The model under review builds one solid part; all positions refer to its coordinate system, in mm. A direction names the side the tool comes from. Give positions to 0.01 mm unless a question says otherwise; leave off trailing zeros. Write each loop counter-clockwise with the first axis right and the second up, starting at its lowest first coordinate (ties: lowest second). Pieces come first, ordered by that corner, then holes. Notation, with made-up numbers: (54, 88.25) -> (82, 88.25) arc R18 cw to (82, 110.25) -> close; hole circle Ø5 at (12.25, 55.25). An arc over 180 degrees is marked (long way). Use CSV: the item, a comma, the result in double quotes.
```python
from build123d import *

# Parameters (mm, degrees)
FASE1_SIZE                                 = 1
F_3_1_3_1_DURCHMESSER_BOHRUNG1_D           = 3.1
F_3_1_3_1_DURCHMESSER_BOHRUNG1_DEPTH       = 15
F_3_1_3_1_DURCHMESSER_BOHRUNG1_CSINK_D     = 3.15
F_3_1_3_1_DURCHMESSER_BOHRUNG1_CSINK_ANGLE = 90
F_3_1_3_1_DURCHMESSER_BOHRUNG1_TIP         = 0.931333959
SCHNITT_LINEAR_AUSTRAGEN1_REACH            = 43.006
SKIZZE5_R                                  = 3
FASE2_SIZE                                 = 1.5


with BuildPart() as part:
    # Skizze1 → Rotation1 (revolve)
    with BuildSketch(Plane.XY, mode=Mode.PRIVATE) as rotation1_sk:
        Polygon((7, 0), (27.5, 0), (27.5, 5.5), (23, 5.5), (23, 6), (19.9, 6), (19.9, 13), (10.6, 13), (10.6, 8), (7, 8), align=None)
    revolve(rotation1_sk.sketch.rotate(Axis((0, 0, 0), (0, -1, 0)), 90), axis=Axis((0, 0, 0), (0, -1, 0)))

    # Fase1
    fase1_edges = [part.edges().sort_by_distance(p)[0] for p in [
        (0, 13, -19.9),
        (0, 13, -10.6),
    ]]
    chamfer(fase1_edges, length=FASE1_SIZE)

    # Ø3.1 (3.1) Durchmesser Bohrung1
    with Locations(Plane(origin=(0, 0, 0), x_dir=(-1, 0, 0), z_dir=(0, -1, 0))):
        with Locations((-16.02146997, 9.25), (0, 18.5), (16.02146997, 9.25), (16.02146997, -9.25), (0, -18.5), (-16.02146997, -9.25)):
            CounterSinkHole(F_3_1_3_1_DURCHMESSER_BOHRUNG1_D / 2, F_3_1_3_1_DURCHMESSER_BOHRUNG1_CSINK_D / 2, depth=F_3_1_3_1_DURCHMESSER_BOHRUNG1_DEPTH, counter_sink_angle=F_3_1_3_1_DURCHMESSER_BOHRUNG1_CSINK_ANGLE)
            with Locations((0, 0, -(F_3_1_3_1_DURCHMESSER_BOHRUNG1_DEPTH + F_3_1_3_1_DURCHMESSER_BOHRUNG1_TIP / 2))):  # 118° drill point
                Cone(0, F_3_1_3_1_DURCHMESSER_BOHRUNG1_D / 2, F_3_1_3_1_DURCHMESSER_BOHRUNG1_TIP, mode=Mode.SUBTRACT)

    # Schnitt-Linear austragen1: up to this face of the body (flat: up to its plane)
    schnitt_linear_austragen1_end = Plane(part.part.faces().sort_by_distance((0, 5.5, -26.722182541))[0])
    # Skizze5 → Schnitt-Linear austragen1 (cut, up to the picked face)
    with BuildSketch(Plane(origin=(0, 13, 0), x_dir=(1, 0, 0), z_dir=(0, 1, 0)), mode=Mode.PRIVATE) as schnitt_linear_austragen1_sk1:
        with Locations(Location((0, 18.5, 0), (0, 0, 3.077902124))):
            Circle(SKIZZE5_R)
    schnitt_linear_austragen1_tool1 = split(extrude(schnitt_linear_austragen1_sk1.sketch, amount=-SCHNITT_LINEAR_AUSTRAGEN1_REACH, mode=Mode.PRIVATE), bisect_by=schnitt_linear_austragen1_end, keep=Keep.BOTH, mode=Mode.PRIVATE)
    # Skizze5 → Schnitt-Linear austragen1 (cut, up to the picked face)
    with BuildSketch(Plane(origin=(0, 13, 0), x_dir=(1, 0, 0), z_dir=(0, 1, 0)), mode=Mode.PRIVATE) as schnitt_linear_austragen1_sk2:
        with Locations(Location((16.02146997, 9.25, 0), (0, 0, 303.077902124))):
            Circle(SKIZZE5_R)
    schnitt_linear_austragen1_tool2 = split(extrude(schnitt_linear_austragen1_sk2.sketch, amount=-SCHNITT_LINEAR_AUSTRAGEN1_REACH, mode=Mode.PRIVATE), bisect_by=schnitt_linear_austragen1_end, keep=Keep.BOTH, mode=Mode.PRIVATE)
    # Skizze5 → Schnitt-Linear austragen1 (cut, up to the picked face)
    with BuildSketch(Plane(origin=(0, 13, 0), x_dir=(1, 0, 0), z_dir=(0, 1, 0)), mode=Mode.PRIVATE) as schnitt_linear_austragen1_sk3:
        with Locations(Location((16.02146997, -9.25, 0), (0, 0, 263.781086479))):
            Circle(SKIZZE5_R)
    schnitt_linear_austragen1_tool3 = split(extrude(schnitt_linear_austragen1_sk3.sketch, amount=-SCHNITT_LINEAR_AUSTRAGEN1_REACH, mode=Mode.PRIVATE), bisect_by=schnitt_linear_austragen1_end, keep=Keep.BOTH, mode=Mode.PRIVATE)
    # Skizze5 → Schnitt-Linear austragen1 (cut, up to the picked face)
    with BuildSketch(Plane(origin=(0, 13, 0), x_dir=(1, 0, 0), z_dir=(0, 1, 0)), mode=Mode.PRIVATE) as schnitt_linear_austragen1_sk4:
        with Locations(Location((0, -18.5, 0), (0, 0, 336.2189135))):
            Circle(SKIZZE5_R)
    schnitt_linear_austragen1_tool4 = split(extrude(schnitt_linear_austragen1_sk4.sketch, amount=-SCHNITT_LINEAR_AUSTRAGEN1_REACH, mode=Mode.PRIVATE), bisect_by=schnitt_linear_austragen1_end, keep=Keep.BOTH, mode=Mode.PRIVATE)
    # Skizze5 → Schnitt-Linear austragen1 (cut, up to the picked face)
    with BuildSketch(Plane(origin=(0, 13, 0), x_dir=(1, 0, 0), z_dir=(0, 1, 0)), mode=Mode.PRIVATE) as schnitt_linear_austragen1_sk5:
        with Locations(Location((-16.02146997, -9.25, 0), (0, 0, 276.2189135))):
            Circle(SKIZZE5_R)
    schnitt_linear_austragen1_tool5 = split(extrude(schnitt_linear_austragen1_sk5.sketch, amount=-SCHNITT_LINEAR_AUSTRAGEN1_REACH, mode=Mode.PRIVATE), bisect_by=schnitt_linear_austragen1_end, keep=Keep.BOTH, mode=Mode.PRIVATE)
    # Skizze5 → Schnitt-Linear austragen1 (cut, up to the picked face)
    with BuildSketch(Plane(origin=(0, 13, 0), x_dir=(1, 0, 0), z_dir=(0, 1, 0)), mode=Mode.PRIVATE) as schnitt_linear_austragen1_sk6:
        with Locations(Location((-16.02146997, 9.25, 0), (0, 0, 236.922097816))):
            Circle(SKIZZE5_R)
    schnitt_linear_austragen1_tool6 = split(extrude(schnitt_linear_austragen1_sk6.sketch, amount=-SCHNITT_LINEAR_AUSTRAGEN1_REACH, mode=Mode.PRIVATE), bisect_by=schnitt_linear_austragen1_end, keep=Keep.BOTH, mode=Mode.PRIVATE)
    add(schnitt_linear_austragen1_tool1.solids().sort_by(Axis((0, 13, -18.5), (0, -1, 0)))[0], mode=Mode.SUBTRACT)
    add(schnitt_linear_austragen1_tool2.solids().sort_by(Axis((16.02147, 13, -9.25), (0, -1, 0)))[0], mode=Mode.SUBTRACT)
    add(schnitt_linear_austragen1_tool3.solids().sort_by(Axis((16.02147, 13, 9.25), (0, -1, 0)))[0], mode=Mode.SUBTRACT)
    add(schnitt_linear_austragen1_tool4.solids().sort_by(Axis((0, 13, 18.5), (0, -1, 0)))[0], mode=Mode.SUBTRACT)
    add(schnitt_linear_austragen1_tool5.solids().sort_by(Axis((-16.02147, 13, 9.25), (0, -1, 0)))[0], mode=Mode.SUBTRACT)
    add(schnitt_linear_austragen1_tool6.solids().sort_by(Axis((-16.02147, 13, -9.25), (0, -1, 0)))[0], mode=Mode.SUBTRACT)

    # Fase2
    # the kernel refuses this chamfer: 1.5 mm, written as the material it takes off along each edge
    with BuildSketch(Plane(origin=(0, 5.5, -18.5), x_dir=(1, 0, 0), z_dir=(0, 0, 1))) as fase2_piece_1_section:
        Polygon((1.55 + FASE2_SIZE, 0), (1.55, -FASE2_SIZE), (1.55, 0), align=None)
    fase2_piece_1 = revolve(axis=Axis((0, 5.5, -18.5), (0, 1, 0)), mode=Mode.PRIVATE)
    fase2_piece_1 = fase2_piece_1 & Plane(origin=(0, 4.721521587, -18.5), x_dir=(0.9985574532138488, 0, -0.053693692656328715), z_dir=(0, 1, 0)) * Cylinder(3, 13, mode=Mode.PRIVATE)
    add(fase2_piece_1, mode=Mode.SUBTRACT)
    with BuildSketch(Plane(origin=(16.02146997, 5.5, -9.25), x_dir=(1, 0, 0), z_dir=(0, 0, 1))) as fase2_piece_2_section:
        Polygon((1.55 + FASE2_SIZE, 0), (1.55, -FASE2_SIZE), (1.55, 0), align=None)
    fase2_piece_2 = revolve(axis=Axis((16.02146997, 5.5, -9.25), (0, 1, 0)), mode=Mode.PRIVATE)
    fase2_piece_2 = fase2_piece_2 & Plane(origin=(16.02146997, 4.721521587, -9.25), x_dir=(0.5457788284702986, 0, 0.83792927529332), z_dir=(0, 1, 0)) * Cylinder(3, 13, mode=Mode.PRIVATE)
    add(fase2_piece_2, mode=Mode.SUBTRACT)
    with BuildSketch(Plane(origin=(16.02146997, 5.5, 9.25), x_dir=(1, 0, 0), z_dir=(0, 0, 1))) as fase2_piece_3_section:
        Polygon((1.55 + FASE2_SIZE, 0), (1.55, -FASE2_SIZE), (1.55, 0), align=None)
    fase2_piece_3 = revolve(axis=Axis((16.02146997, 5.5, 9.25), (0, 1, 0)), mode=Mode.PRIVATE)
    fase2_piece_3 = fase2_piece_3 & Plane(origin=(16.02146997, 4.721521587, 9.25), x_dir=(-0.10832752224481851, 0, 0.9941152588730838), z_dir=(0, 1, 0)) * Cylinder(3, 13, mode=Mode.PRIVATE)
    add(fase2_piece_3, mode=Mode.SUBTRACT)
    with BuildSketch(Plane(origin=(0, 5.5, 18.5), x_dir=(1, 0, 0), z_dir=(0, 0, 1))) as fase2_piece_4_section:
        Polygon((1.55 + FASE2_SIZE, 0), (1.55, -FASE2_SIZE), (1.55, 0), align=None)
    fase2_piece_4 = revolve(axis=Axis((0, 5.5, 18.5), (0, 1, 0)), mode=Mode.PRIVATE)
    fase2_piece_4 = fase2_piece_4 & Plane(origin=(0, 4.721521587, 18.5), x_dir=(0.915092829448447, 0, 0.4032432435789042), z_dir=(0, 1, 0)) * Cylinder(3, 13, mode=Mode.PRIVATE)
    add(fase2_piece_4, mode=Mode.SUBTRACT)
    with BuildSketch(Plane(origin=(-16.02146997, 5.5, -9.25), x_dir=(1, 0, 0), z_dir=(0, 0, 1))) as fase2_piece_5_section:
        Polygon((1.55 + FASE2_SIZE, 0), (1.55, -FASE2_SIZE), (1.55, 0), align=None)
    fase2_piece_5 = revolve(axis=Axis((-16.02146997, 5.5, -9.25), (0, 1, 0)), mode=Mode.PRIVATE)
    fase2_piece_5 = fase2_piece_5 & Plane(origin=(-16.02146997, 4.721521587, -9.25), x_dir=(-0.5457788293477767, 0, 0.8379292747217814), z_dir=(0, 1, 0)) * Cylinder(3, 13, mode=Mode.PRIVATE)
    add(fase2_piece_5, mode=Mode.SUBTRACT)
    with BuildSketch(Plane(origin=(-16.02146997, 5.5, 9.25), x_dir=(1, 0, 0), z_dir=(0, 0, 1))) as fase2_piece_6_section:
        Polygon((1.55 + FASE2_SIZE, 0), (1.55, -FASE2_SIZE), (1.55, 0), align=None)
    fase2_piece_6 = revolve(axis=Axis((-16.02146997, 5.5, 9.25), (0, 1, 0)), mode=Mode.PRIVATE)
    fase2_piece_6 = fase2_piece_6 & Plane(origin=(-16.02146997, 4.721521587, 9.25), x_dir=(0.10832752188045662, 0, 0.9941152589127878), z_dir=(0, 1, 0)) * Cylinder(3, 13, mode=Mode.PRIVATE)
    add(fase2_piece_6, mode=Mode.SUBTRACT)


solid = part.part
```
Q1. Consider section A-A (z = 0). Write out the cut boundary in (x, y).
Derived:
outline,"(-27.5, 0) -> (-7, 0) -> (-7, 8) -> (-10.6, 8) -> (-10.6, 12) -> (-11.6, 13) -> (-18.9, 13) -> (-19.9, 12) -> (-19.9, 6) -> (-23, 6) -> (-23, 5.5) -> (-27.5, 5.5) -> close; (7, 0) -> (27.5, 0) -> (27.5, 5.5) -> (23, 5.5) -> (23, 6) -> (19.9, 6) -> (19.9, 12) -> (18.9, 13) -> (11.6, 13) -> (10.6, 12) -> (10.6, 8) -> (7, 8) -> close"
Q2. The part is to be moulded in two halves that separate along Z. For faces 1 (the flat face through (-9, 13, 8)), 2 (the cylindrical face through (-0.202, 2.04, -20.037)), 3 (the conical face through (-9.5, 12.73, 16.65)), say which applies: pulls with the +Z half, pulls with the -Z half, needs draft (parallel to the pull), parting line crosses it, or undercut.
Derived:
face 1,"needs draft"
face 2,"undercut"
face 3,"pulls with the +Z half"
Q3. Consider section C-C (z = 9.25). State how many separate pieces and enclosed holes the cut face has, then the cut area to 3 significant figures.
Derived:
separate pieces,"3"
enclosed holes,"0"
area,"390 mm2"
Q4. Insertion check: pin 1 (1.5 mm diameter, centred on x = -2.5, y = 3, fed in from +Z); pin 2 (2 mm diameter, centred on y = 1.5, z = -19.5, fed in from +X); pin 3 (5 mm diameter, centred on y = 5, z = 8, fed in from +X). Each pin has a flat end and moves straight along its axis. Give the tip position at first contact, or say it passes through.
Derived:
pin 1,"stops at z = 27.44"
pin 2,"stops at x = 20.35"
pin 3,"stops at x = 26.94"
Q5. Consider section B-B (y = 11). Write out the cut boundary in (x, z).
Derived:
outline,"(-18.44, -7.48) arc R3 cw (long way) to (-15.7, -12.23) arc R19.9 ccw to (-2.75, -19.71) arc R3 cw (long way) to (2.75, -19.71) arc R19.9 ccw to (15.7, -12.23) arc R3 cw (long way) to (18.44, -7.48) arc R19.9 ccw to (18.44, 7.48) arc R3 cw (long way) to (15.7, 12.23) arc R19.9 ccw to (2.75, 19.71) arc R3 cw (long way) to (-2.75, 19.71) arc R19.9 ccw to (-15.7, 12.23) arc R3 cw (long way) to (-18.44, 7.48) arc R19.9 ccw to start; hole circle Ø21.2 at (0, 0)"
Q6. Machinability: for faces 4 (the cylindrical face through (6.45, 9.97, -8.41)), 5 (the cylindrical face through (10.04, 9.04, 17.18)), 6 (the cylindrical face through (-10.04, 9.04, -17.18)), 7 (the cylindrical face through (-19.9, 9, 0.1)), 8 (the cylindrical face through (-0.202, 2.04, 16.963)), which of the approach directions +Z, -Z, +X, -X, +Y, -Y give a long, thin tool a straight path to every point of the face, cutting with its end or side? Answer none if there is none.
Derived:
face 4,"+Y"
face 5,"+Z, +X, +Y"
face 6,"-Z, -X, +Y"
face 7,"-X, +Y"
face 8,"+Y, -Y"
Q7. To check wall thickness, follow probe 1 along Z at (x, y) = (16.5, 4.5); probe 2 along X at (y, z) = (2.25, -9.25); probe 3 along X at (y, z) = (4.75, -10). State the ranges of each line that lie inside material, in increasing order.
Derived:
probe 1,"z = -22 to -11.24, -7.26 to 7.26, 11.24 to 22"
probe 2,"x = -25.9 to -17.57, -14.47 to 14.47, 17.57 to 25.9"
probe 3,"x = -25.62 to -18.2, -13.85 to 13.85, 18.2 to 25.62"
